Geometry: final body of the model. Coordinates: model frame, mm. Face numbers are marked on the shaded views. A direction names the side the tool comes from. Round coordinates to 2 decimals unless told otherwise and drop trailing zeros. Write each loop counter-clockwise with the first axis right and the second up, starting at its lowest first coordinate (ties: lowest second). Pieces come first, ordered by that corner, then holes. Notation, with made-up numbers: (85.25, 38.5) -> (138.25, 38.5) arc R10 cw to (138.25, 49.5) -> close; hole circle Ø2 at (38.5, 35.25). An arc over 180 degrees is marked (long way). One line per item, written item: value. Start each with the question number.
Autodesk Inventor part; units mm, degrees
ref_plane "dia1_XY" through (0, 3.175, 0) normal (1, 0, 0) x (0, 0, -1)
ref_plane "dia1_YZ" through (0, 3.175, 0) normal (0, 0, -1) x (0, 1, 0)
ref_plane "dia1_ZX" through (0, 3.175, 0) normal (0, 1, 0) x (1, 0, 0)
sketch "Sketch_1" plane through (0, 0, 0) normal (0, 0, 1) x (1, 0, 0)
  line L0 (110.4646, 0) -> (0, 0)
  line L1 (0, 0) -> (0, 3.175)
  line L2 (0, 3.175) -> (73.025, 3.175)
  line L3 (73.025, 3.175) -> (73.025, 9.6203)
  line L4 (73.025, 9.6203) -> (110.4646, 9.6203)
  line L5 (110.4646, 9.6203) -> (110.4646, 0)
  line L6 (110.4646, 0) -> (0, 0)
revolve "Revolution1" add sketch "Sketch_1" angle 360 about axis through (110.4646, 0, 0) along (1, 0, 0)
sketch "Sketch_3" plane through (0, 0, 0) normal (0, 0, 1) x (1, 0, 0)
  line L0 (0, 0) -> (-12.7, 0)
  line L1 (-12.7, 0) -> (-12.7, 2.634)
  line L2 (-12.7, 2.634) -> (-12.159, 3.175)
  line L3 (-12.159, 3.175) -> (0, 3.175)
  line L4 (0, 3.175) -> (0, 0)
  line L5 (0, 0) -> (-12.7, 0)
revolve "Revolution2" add sketch "Sketch_3" angle 360 about axis through (0, 0, 0) along (1, 0, 0)
thread "Thread1"
sketch "Sketch_30" plane through (0, 0, 0) normal (0, 0, 1) x (1, 0, 0)
  line L0 (0, 0) -> (-0.254, 0)
  line L1 (-0.254, 2.921) -> (0, 2.921)
  line L2 (0, 2.921) -> (0, 3.429)
  line L3 (0, 3.429) -> (-0.254, 3.429)
  line L4 (-0.254, 3.429) -> (-0.254, 2.921)
revolve "Revolution3" cut sketch "Sketch_30" angle 360 about axis through (0, 0, 0) along (1, 0, 0)
ref_plane "dia1_XY" through (0, 3.175, 0) normal (1, 0, 0) x (0, 0, -1)
ref_plane "dia1_YZ" through (0, 3.175, 0) normal (0, 0, -1) x (0, 1, 0)
ref_plane "dia1_ZX" through (0, 3.175, 0) normal (0, 1, 0) x (1, 0, 0)
ref_plane "dia12_XY" through (0, 0, 10.2235) normal (1, 0, 0) x (0, 0, -1)
ref_plane "dia12_YZ" through (0, 0, 10.2235) normal (0, 0, -1) x (0, 1, 0)
ref_plane "dia12_ZX" through (0, 0, 10.2235) normal (0, 1, 0) x (1, 0, 0)
ref_plane "dia2_XY" through (0, -3.175, 0) normal (1, 0, 0) x (0, 0, -1)
ref_plane "dia2_YZ" through (0, -3.175, 0) normal (0, 0, -1) x (0, 1, 0)
ref_plane "dia2_ZX" through (0, -3.175, 0) normal (0, 1, 0) x (1, 0, 0)
ref_plane "dia22_XY" through (0, 0, -10.2235) normal (1, 0, 0) x (0, 0, -1)
ref_plane "dia22_YZ" through (0, 0, -10.2235) normal (0, 0, -1) x (0, 1, 0)
ref_plane "dia22_ZX" through (0, 0, -10.2235) normal (0, 1, 0) x (1, 0, 0)
ref_plane "rl1_XY" through (-12.7, 0, 0) normal (1, 0, 0) x (0, 0, -1)
ref_plane "rl1_YZ" through (-12.7, 0, 0) normal (0, 0, -1) x (0, 1, 0)
ref_plane "rl1_ZX" through (-12.7, 0, 0) normal (0, 1, 0) x (1, 0, 0)
ref_plane "rl2_XY" through (0, 0, 0) normal (1, 0, 0) x (0, 0, -1)
ref_plane "rl2_YZ" through (0, 0, 0) normal (0, 0, -1) x (0, 1, 0)
ref_plane "rl2_ZX" through (0, 0, 0) normal (0, 1, 0) x (1, 0, 0)
ref_plane "rod_cp_XY" through (0, 0, 0) normal (1, 0, 0) x (0, 0, -1)
ref_plane "rod_cp_YZ" through (0, 0, 0) normal (0, 0, -1) x (0, 1, 0)
ref_plane "rod_cp_ZX" through (0, 0, 0) normal (0, 1, 0) x (1, 0, 0)
ref_plane "thd1_XY" through (-12.7, 3.175, 0) normal (1, 0, 0) x (0, 0, -1)
ref_plane "thd1_YZ" through (-12.7, 3.175, 0) normal (0, 0, -1) x (0, 1, 0)
ref_plane "thd1_ZX" through (-12.7, 3.175, 0) normal (0, 1, 0) x (1, 0, 0)
ref_plane "thd2_XY" through (-12.7, -3.175, 0) normal (1, 0, 0) x (0, 0, -1)
ref_plane "thd2_YZ" through (-12.7, -3.175, 0) normal (0, 0, -1) x (0, 1, 0)
ref_plane "thd2_ZX" through (-12.7, -3.175, 0) normal (0, 1, 0) x (1, 0, 0)
ref_plane "to_rod_clevis_XY" through (-16.764, 0, 0) normal (1, 0, 0) x (0, 0, -1)
ref_plane "to_rod_clevis_YZ" through (-16.764, 0, 0) normal (0, 0, -1) x (0, 1, 0)
ref_plane "to_rod_clevis_ZX" through (-16.764, 0, 0) normal (0, 1, 0) x (1, 0, 0)
properties part number "C-0420000_rod"
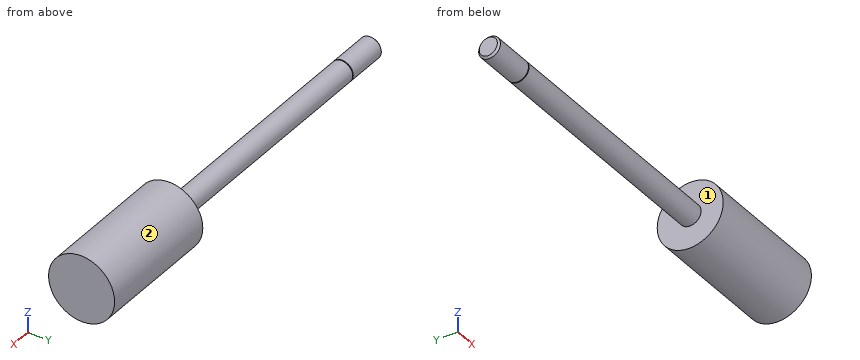
(1) Line query: probe 1 along X at (y, z) = (3.5, 8) (3 decimals); probe 2 along Y at (x, z) = (80.5, -0.25); probe 3 along X at (y, z) = (-2, -2). Output: solid intervals per line, ascending.
(2) Section query C-C (x = 16). Output: boundary loops of the cut face in (y, z) (3 decimals), and give its area (3 significant figures).
(3) Section query A-A (y = 0). Output: boundary loops of the cut face in (x, z) (3 decimals).
(4) Set-up query: the marked faces 1 and 2. Return all of +Z, -Z, +X, -X, +Y, -Y with unobstructed straight access to the full face (end or side cutting, diameter ignored); none if empty.
(5) Section query D-D (x = 83). Output: boundary loops of the cut face in (y, z), and give its area (3 significant figures).
(6) Pin query (flat end, axial travel): pin 1 (8 mm diameter, centred on y = -7.5, z = -2.5, fed in from -X) (3 decimals); pin 2 (8 mm diameter, centred on x = 23, y = -2.5, fed in from -Z) (3 decimals); pin 3 (8 mm diameter, centred on x = 77, y = 5.5, fed in from -Z). Return the tip coordinate at first contact, or that it passes through.
Results list:
1. probe 1: x = 73.025 to 110.465
1. probe 2: y = -9.62 to 9.62
1. probe 3: x = -12.51 to 110.46
2. outline: circle Ø6.35 at (0, 0)
2. area: 31.7 mm^2
3. outline: (-12.7, -2.634) -> (-12.159, -3.175) -> (-0.254, -3.175) -> (-0.254, -2.921) -> (0, -2.921) -> (0, -3.175) -> (73.025, -3.175) -> (73.025, -9.62) -> (110.465, -9.62) -> (110.465, 9.62) -> (73.025, 9.62) -> (73.025, 3.175) -> (0, 3.175) -> (0, 2.921) -> (-0.254, 2.921) -> (-0.254, 3.175) -> (-12.159, 3.175) -> (-12.7, 2.634) -> close
4. face 1: -X
4. face 2: +X, -X
5. outline: circle Ø19.24 at (0, 0)
5. area: 291 mm^2
6. pin 1: stops at x = 73.025
6. pin 2: stops at z = -3.175
6. pin 3: stops at z = -9.5
